```python
from build123d import *

# Parameters (mm, degrees)
SKETCH3_R           = 2.05
BOSS_EXTRUDE2_DEPTH = 3.175
FILLET1_R           = 10
FILLET2_R           = 1
SKETCH6_R           = 2.05
CUT_EXTRUDE3_DEPTH  = 3.18


with BuildPart() as part:
    # Sketch3 → Boss-Extrude2 (new body)
    with BuildSketch(Plane(origin=(0, 0, 0), x_dir=(1, 0, 0), z_dir=(0, 1, 0))):
        Polygon((-184, -11.5875), (-148, -47.5875), (-108, -47.5875), (-94, -33.5875), (94, -33.5875), (108, -47.5875), (148, -47.5875), (184, -11.5875), (184, 59.5875), (-184, 59.5875), align=None)
        with Locations(Location((-128, -11.5875, 0), (0, 0, 270))):
            Circle(SKETCH3_R, mode=Mode.SUBTRACT)
        with Locations(Location((128, -11.5875, 0), (0, 0, 90))):
            Circle(SKETCH3_R, mode=Mode.SUBTRACT)
    extrude(amount=BOSS_EXTRUDE2_DEPTH)

    # Fillet1
    fillet1_edges = [part.edges().sort_by_distance(p)[0] for p in [
        (184, 1.5875, 11.5875),
        (148, 1.5875, 47.5875),
        (108, 1.5875, 47.5875),
        (94, 1.5875, 33.5875),
        (-94, 1.5875, 33.5875),
        (-108, 1.5875, 47.5875),
        (-148, 1.5875, 47.5875),
        (-184, 1.5875, 11.5875),
    ]]
    fillet(fillet1_edges, radius=FILLET1_R)

    # Fillet2
    fillet2_edges = [part.edges().sort_by_distance(p)[0] for p in [
        (184, 1.5875, -59.5875),
        (-184, 1.5875, -59.5875),
    ]]
    fillet(fillet2_edges, radius=FILLET2_R)

    # Sketch6 → Cut-Extrude3 (cut)
    with BuildSketch(Plane(origin=(0, 3.175, 0), x_dir=(1, 0, 0), z_dir=(0, 1, 0))):
        with Locations(Location((-176, 48.4125, 0), (0, 0, 270))):
            Circle(SKETCH6_R)
        with Locations(Location((-160, 48.4125, 0), (0, 0, 270))):
            Circle(SKETCH6_R)
        with Locations(Location((-144, 48.4125, 0), (0, 0, 270))):
            Circle(SKETCH6_R)
        with Locations(Location((-128, 48.4125, 0), (0, 0, 270))):
            Circle(SKETCH6_R)
        with Locations(Location((-112, 48.4125, 0), (0, 0, 270))):
            Circle(SKETCH6_R)
        with Locations(Location((-96, 48.4125, 0), (0, 0, 270))):
            Circle(SKETCH6_R)
        with Locations(Location((-80, 48.4125, 0), (0, 0, 270))):
            Circle(SKETCH6_R)
        with Locations(Location((-64, 48.4125, 0), (0, 0, 270))):
            Circle(SKETCH6_R)
        with Locations(Location((-48, 48.4125, 0), (0, 0, 270))):
            Circle(SKETCH6_R)
        with Locations(Location((-32, 48.4125, 0), (0, 0, 270))):
            Circle(SKETCH6_R)
        with Locations(Location((-16, 48.4125, 0), (0, 0, 270))):
            Circle(SKETCH6_R)
        with Locations(Location((0, 48.4125, 0), (0, 0, 270))):
            Circle(SKETCH6_R)
        with Locations(Location((16, 48.4125, 0), (0, 0, 270))):
            Circle(SKETCH6_R)
        with Locations(Location((32, 48.4125, 0), (0, 0, 270))):
            Circle(SKETCH6_R)
        with Locations(Location((48, 48.4125, 0), (0, 0, 270))):
            Circle(SKETCH6_R)
        with Locations(Location((64, 48.4125, 0), (0, 0, 270))):
            Circle(SKETCH6_R)
        with Locations(Location((80, 48.4125, 0), (0, 0, 270))):
            Circle(SKETCH6_R)
        with Locations(Location((96, 48.4125, 0), (0, 0, 270))):
            Circle(SKETCH6_R)
        with Locations(Location((112, 48.4125, 0), (0, 0, 270))):
            Circle(SKETCH6_R)
        with Locations(Location((128, 48.4125, 0), (0, 0, 270))):
            Circle(SKETCH6_R)
        with Locations(Location((144, 48.4125, 0), (0, 0, 270))):
            Circle(SKETCH6_R)
        with Locations(Location((160, 48.4125, 0), (0, 0, 270))):
            Circle(SKETCH6_R)
        with Locations(Location((176, 48.4125, 0), (0, 0, 270))):
            Circle(SKETCH6_R)
        with Locations(Location((175.986011582, 32.412506115, 0), (0, 0, 270))):
            Circle(SKETCH6_R)
        with Locations(Location((175.972023163, 16.41251223, 0), (0, 0, 270))):
            Circle(SKETCH6_R)
        with Locations(Location((-176.013988418, 32.412506115, 0), (0, 0, 270))):
            Circle(SKETCH6_R)
        with Locations(Location((-176.027976837, 16.41251223, 0), (0, 0, 270))):
            Circle(SKETCH6_R)
    extrude(amount=-CUT_EXTRUDE3_DEPTH, mode=Mode.SUBTRACT)


solid = part.part
```
Model file for the job. Use its own axes, mm. A direction names the side the tool comes from. Give positions to 0.01 mm unless a question says otherwise; leave off trailing zeros. Order: outer loops, then holes, each group sorted by start corner. A loop starts at its lowest first (then second) coordinate and runs counter-clockwise, first axis right, second up.
1) Pin check, flat tip, straight feed: pin 1 (2.5 mm diameter, centred on x = -80, z = -48.41, fed in from -Y). Stop position of the tip, or through.
2) 3-axis set-ups, long thin cutter, end or side, ignore diameter. For faces 4 (the flat face through (100.94, 1.57, 40.53)), 5 (the flat face through (-166.21, 1.57, 29.38)): which of +Z, -Z, +X, -X, +Y, -Y reach the whole face in a straight line?
3) Wall check: probe 1 along Z at (x, y) = (128, 1.1); probe 2 along X at (y, z) = (3.05, 14.5); probe 3 along X at (y, z) = (2.3, 8). Give the ranges that are in metal, low to high.
4) Mould opens along X. For faces 1 (the flat face through (-3, 0, -7)), 2 (the flat face through (-101.057, 1.565, 40.644)), 3 (the flat face through (165.79, 1.57, 29.8)) say: +X half, -X half, draft (parallel to the pull), parting line (faces both ways), or undercut.
5) Saw through at C-C, the plane z = 19. Write the cut outline in (x, y) (1 decimal).
6) Saw through at A-A, the plane y = 1.25. Count the separate pieces of the cut face and the enclosed holes in it, then the cut area to 3 significant figures.
7) Saw through at B-B, the plane x = 5.5. Write the cut outline in (y, z) (1 decimal), then the cut area to 3 significant figures.
Computed:
1. pin 1: passes through
2. face 4: +Z, +Y, -Y
2. face 5: +Z, -X, +Y, -Y
3. probe 1: z = -59.59 to -50.46, -46.36 to 9.54, 13.64 to 47.59
3. probe 2: x = -181.09 to 181.09
3. probe 3: x = -183.98 to 183.98
4. face 1: draft
4. face 2: undercut
4. face 3: +X half
5. outline: (-176.6, 0) - (176.6, 0) - (176.6, 3.2) - (-176.6, 3.2) - close
6. separate pieces: 1
6. enclosed holes: 29
6. area: 34,900 mm2
7. outline: (0, -59.6) - (3.2, -59.6) - (3.2, 33.6) - (0, 33.6) - close
7. area: 296 mm2
